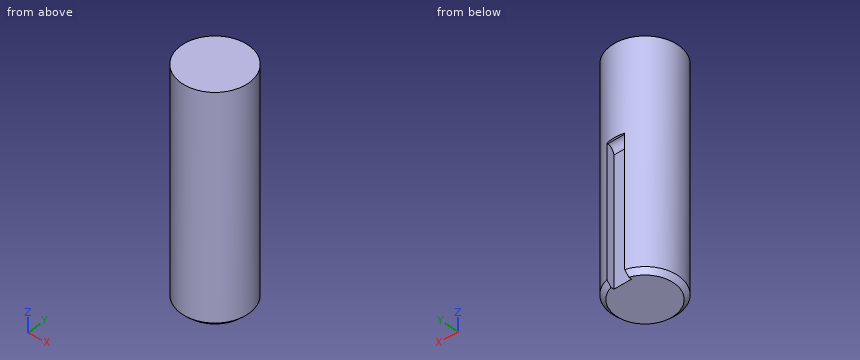
```python
from build123d import *

# Parameters (mm, degrees)
SKETCH1_R           = 15
BOSS_EXTRUDE1_DEPTH = 100
CHAMFER1_SIZE       = 2
SKETCH3_W           = 8
SKETCH3_H           = 60
CUT_EXTRUDE1_DEPTH  = 4
FILLET1_R           = 3
ESCALA1_SCALE       = 0.5


with BuildPart() as part:
    # Sketch1 → Boss-Extrude1 (new body)
    with BuildSketch(Plane.XY):
        Circle(SKETCH1_R)
    extrude(amount=BOSS_EXTRUDE1_DEPTH)

    # Chamfer1
    chamfer1_edges = [part.edges().sort_by_distance(p)[0] for p in [
        (-15, 0, 0),
    ]]
    chamfer(chamfer1_edges, length=CHAMFER1_SIZE)

    # Sketch3 → Cut-Extrude1 (cut)
    with BuildSketch(Plane(origin=(0, 15, 100), x_dir=(1, 0, 0), z_dir=(0, 1, 0))):
        with Locations((0, 70)):
            Rectangle(SKETCH3_W, SKETCH3_H)
    extrude(amount=-CUT_EXTRUDE1_DEPTH, mode=Mode.SUBTRACT)

    # Fillet1
    fillet1_edges = [part.edges().sort_by_distance(p)[0] for p in [
        (0, 11, 60),
    ]]
    fillet(fillet1_edges, radius=FILLET1_R)


with BuildPart() as part_1:
    # Escala1: scaled about (0, -0.338706131, 50.653578584)
    add(part.part.scale(ESCALA1_SCALE).moved(Location((0, -0.169353066, 25.326789292))))


solid = part_1.part
```
Source: CAD feature listing. Evaluate the final solid. Frame: model axes, mm. Round coordinates to 2 decimals unless told otherwise and drop trailing zeros. Write each loop counter-clockwise with the first axis right and the second up, starting at its lowest first coordinate (ties: lowest second). Pieces come first, ordered by that corner, then holes. Notation, with made-up numbers: M 71,18 L 124,18 A22 ccw 124,33 Z; hole C -7.5,80.5 d2. An arc over 180 degrees is marked long. Answer as a JSON object with one key per item and string values. Group by question number.
(1) Section query A-A on x = 0. Output: boundary loops of the cut face in (y, z).
(2) Section query C-C on z = 60. Output: boundary loops of the cut face in (x, y).
(3) First-contact query: pin 1 (0.5 mm diameter, centred on y = 6, z = 34.5, fed in from +X); pin 2 (2 mm diameter, centred on x = 0.5, z = 42.5, fed in from +Y); pin 3 (8 mm diameter, centred on y = -4.5, z = 58, fed in from +X). Flat tips, straight axial feed; report the tip coordinate or a pass-through.
(4) Section query B-B on z = 48. Output: boundary loops of the cut face in (x, y).
(5) Ray query, line 1 (Y direction, x = 2.75, z = 33); line 2 (Z direction, x = -6.25, y = 3); line 3 (X direction, y = -6.25, z = 34). Return the intervals inside material, ascending. Write a range as [from, to].
Computed values:
{
 "1": {"outline": "M -7.67,26.33 L -6.67,25.33 L 5.33,25.33 L 5.33,53.83 A1.5 cw 6.83,55.33 L 7.33,55.33 L 7.33,75.33 L -7.67,75.33 Z"},
 "2": {"outline": "C 0,-0.17 d15"},
 "3": {"pin 1": "x = 4.61", "pin 2": "y = 5.33", "pin 3": "x = 7.49"},
 "4": {"outline": "M -2,5.33 L -2,7.06 A7.5 ccw long 2,7.06 L 2,5.33 Z"},
 "5": {"line 1": "[-7.15, 6.81]", "line 2": "[25.83, 75.33]", "line 3": "[-4.39, 4.39]"}
}
